from build123d import *

# Parameters (mm, degrees)
PARED_DEPTH             = 23
CONECTORES_REACH        = 154.052
CROQUIS2_W              = 16
CROQUIS2_H              = 13
CROQUIS2_W_2            = 10
CROQUIS2_H_2            = 4
BASE_START              = -1.12
BASE_FRENTE_DEPTH       = 1.12
LUCES_REACH             = 153.399
CROQUIS3_R              = 1.5
CROQUIS3_R_2            = 2.5
SALIENTE_EXTRUIR1_START = 12
CROQUIS3_3_R            = 2.3
CROQUIS3_3_R_2          = 1.5
SALIENTE_EXTRUIR1_DEPTH = 12
SALIENTE_EXTRUIR2_START = 9
CROQUIS3_4_R            = 3.3
CROQUIS3_4_R_2          = 2.5
SALIENTE_EXTRUIR2_DEPTH = 9
SALIENTE_EXTRUIR3_START = 6
CROQUIS3_5_R            = 2.3
CROQUIS3_5_R_2          = 1.5
SALIENTE_EXTRUIR3_DEPTH = 6


with BuildPart() as part:
    # Croquis1 → pared (new body)
    with BuildSketch(Plane.XY):
        with BuildLine():
            Line((3, 61.1), (132, 61.1))
            ThreePointArc((132, 61.1), (135.252691193, 59.752691193), (136.6, 56.5))
            Line((136.6, 56.5), (136.6, 3))
            ThreePointArc((136.6, 3), (135.252691193, -0.252691193), (132, -1.6))
            Line((132, -1.6), (3, -1.6))
            ThreePointArc((3, -1.6), (-0.252691193, -0.252691193), (-1.6, 3))
            Line((-1.6, 3), (-1.6, 56.5))
            ThreePointArc((-1.6, 56.5), (-0.252691193, 59.752691193), (3, 61.1))
        make_face()
        with BuildLine():
            Line((3, 0), (132, 0))
            ThreePointArc((132, 0), (134.121320344, 0.878679656), (135, 3))
            Line((135, 3), (135, 56.5))
            ThreePointArc((135, 56.5), (134.121320344, 58.621320344), (132, 59.5))
            Line((132, 59.5), (3, 59.5))
            ThreePointArc((3, 59.5), (0.878679656, 58.621320344), (0, 56.5))
            Line((0, 56.5), (0, 3))
            ThreePointArc((0, 3), (0.878679656, 0.878679656), (3, 0))
        make_face(mode=Mode.SUBTRACT)
    extrude(amount=PARED_DEPTH)

    # Croquis2 → conectores (cut, up to next)
    with BuildSketch(Plane.XZ.offset(1.6), mode=Mode.PRIVATE) as conectores_sk1:
        with Locations((110, 6.5)):
            Rectangle(CROQUIS2_W, CROQUIS2_H)
    conectores_tool1 = extrude(conectores_sk1.sketch, amount=-CONECTORES_REACH, mode=Mode.PRIVATE) & part.part
    # Croquis2 → conectores (cut, up to next)
    with BuildSketch(Plane.XZ.offset(1.6), mode=Mode.PRIVATE) as conectores_sk2:
        with Locations((95, 12)):
            Rectangle(CROQUIS2_W_2, CROQUIS2_H_2)
    conectores_tool2 = extrude(conectores_sk2.sketch, amount=-CONECTORES_REACH, mode=Mode.PRIVATE) & part.part
    add(conectores_tool1.solids().sort_by_distance((110, -1.6, 6.5))[0], mode=Mode.SUBTRACT)
    add(conectores_tool2.solids().sort_by_distance((95, -1.6, 12))[0], mode=Mode.SUBTRACT)

    # Croquis1<2> → base frente (add)
    with BuildSketch(Plane.XY.offset(BASE_START)):
        with BuildLine():
            Line((3, 61.1), (132, 61.1))
            ThreePointArc((132, 61.1), (135.252691193, 59.752691193), (136.6, 56.5))
            Line((136.6, 56.5), (136.6, 3))
            ThreePointArc((136.6, 3), (135.252691193, -0.252691193), (132, -1.6))
            Line((132, -1.6), (3, -1.6))
            ThreePointArc((3, -1.6), (-0.252691193, -0.252691193), (-1.6, 3))
            Line((-1.6, 3), (-1.6, 56.5))
            ThreePointArc((-1.6, 56.5), (-0.252691193, 59.752691193), (3, 61.1))
        make_face()
    extrude(amount=BASE_FRENTE_DEPTH)

    # Croquis3 → luces (cut, up to next)
    with BuildSketch(Plane.XY, mode=Mode.PRIVATE) as luces_sk1:
        with Locations((130.5, 48)):
            Circle(CROQUIS3_R)
    luces_tool1 = extrude(luces_sk1.sketch, amount=-LUCES_REACH, mode=Mode.PRIVATE) & part.part
    # Croquis3 → luces (cut, up to next)
    with BuildSketch(Plane.XY, mode=Mode.PRIVATE) as luces_sk2:
        with Locations((130.5, 41.5)):
            Circle(CROQUIS3_R)
    luces_tool2 = extrude(luces_sk2.sketch, amount=-LUCES_REACH, mode=Mode.PRIVATE) & part.part
    # Croquis3 → luces (cut, up to next)
    with BuildSketch(Plane.XY, mode=Mode.PRIVATE) as luces_sk3:
        with Locations((130.5, 35)):
            Circle(CROQUIS3_R)
    luces_tool3 = extrude(luces_sk3.sketch, amount=-LUCES_REACH, mode=Mode.PRIVATE) & part.part
    # Croquis3 → luces (cut, up to next)
    with BuildSketch(Plane.XY, mode=Mode.PRIVATE) as luces_sk4:
        with Locations((130.5, 28.5)):
            Circle(CROQUIS3_R)
    luces_tool4 = extrude(luces_sk4.sketch, amount=-LUCES_REACH, mode=Mode.PRIVATE) & part.part
    # Croquis3 → luces (cut, up to next)
    with BuildSketch(Plane.XY, mode=Mode.PRIVATE) as luces_sk5:
        with Locations((130.5, 17.5)):
            Circle(CROQUIS3_R)
    luces_tool5 = extrude(luces_sk5.sketch, amount=-LUCES_REACH, mode=Mode.PRIVATE) & part.part
    # Croquis3 → luces (cut, up to next)
    with BuildSketch(Plane.XY, mode=Mode.PRIVATE) as luces_sk6:
        with Locations((130.5, 11.5)):
            Circle(CROQUIS3_R_2)
    luces_tool6 = extrude(luces_sk6.sketch, amount=-LUCES_REACH, mode=Mode.PRIVATE) & part.part
    # Croquis3 → luces (cut, up to next)
    with BuildSketch(Plane.XY, mode=Mode.PRIVATE) as luces_sk7:
        with Locations((3.5, 15)):
            Circle(CROQUIS3_R)
    luces_tool7 = extrude(luces_sk7.sketch, amount=-LUCES_REACH, mode=Mode.PRIVATE) & part.part
    add(luces_tool1.solids().sort_by_distance((130.5, 48, 0))[0], mode=Mode.SUBTRACT)
    add(luces_tool2.solids().sort_by_distance((130.5, 41.5, 0))[0], mode=Mode.SUBTRACT)
    add(luces_tool3.solids().sort_by_distance((130.5, 35, 0))[0], mode=Mode.SUBTRACT)
    add(luces_tool4.solids().sort_by_distance((130.5, 28.5, 0))[0], mode=Mode.SUBTRACT)
    add(luces_tool5.solids().sort_by_distance((130.5, 17.5, 0))[0], mode=Mode.SUBTRACT)
    add(luces_tool6.solids().sort_by_distance((130.5, 11.5, 0))[0], mode=Mode.SUBTRACT)
    add(luces_tool7.solids().sort_by_distance((3.5, 15, 0))[0], mode=Mode.SUBTRACT)

    # Croquis3<3> → Saliente-Extruir1 (add)
    # profile 1 of 5: a face of its own
    with BuildSketch(Plane.XY.offset(SALIENTE_EXTRUIR1_START)):
        with Locations((130.5, 17.5)):
            Circle(CROQUIS3_3_R)
        with Locations((130.5, 17.5)):
            Circle(CROQUIS3_3_R_2, mode=Mode.SUBTRACT)
    # profile 2 of 5: a face of its own
    with BuildSketch(Plane.XY.offset(SALIENTE_EXTRUIR1_START)):
        with Locations((130.5, 28.5)):
            Circle(CROQUIS3_3_R)
        with Locations((130.5, 28.5)):
            Circle(CROQUIS3_3_R_2, mode=Mode.SUBTRACT)
    # profile 3 of 5: a face of its own
    with BuildSketch(Plane.XY.offset(SALIENTE_EXTRUIR1_START)):
        with Locations((130.5, 35)):
            Circle(CROQUIS3_3_R)
        with Locations((130.5, 35)):
            Circle(CROQUIS3_3_R_2, mode=Mode.SUBTRACT)
    # profile 4 of 5: a face of its own
    with BuildSketch(Plane.XY.offset(SALIENTE_EXTRUIR1_START)):
        with Locations((130.5, 41.5)):
            Circle(CROQUIS3_3_R)
        with Locations((130.5, 41.5)):
            Circle(CROQUIS3_3_R_2, mode=Mode.SUBTRACT)
    # profile 5 of 5: a face of its own
    with BuildSketch(Plane.XY.offset(SALIENTE_EXTRUIR1_START)):
        with Locations((130.5, 48)):
            Circle(CROQUIS3_3_R)
        with Locations((130.5, 48)):
            Circle(CROQUIS3_3_R_2, mode=Mode.SUBTRACT)
    extrude(amount=-SALIENTE_EXTRUIR1_DEPTH)

    # Croquis3<4> → Saliente-Extruir2 (add)
    with BuildSketch(Plane.XY.offset(SALIENTE_EXTRUIR2_START)):
        with Locations((130.5, 11.5)):
            Circle(CROQUIS3_4_R)
        with Locations((130.5, 11.5)):
            Circle(CROQUIS3_4_R_2, mode=Mode.SUBTRACT)
    extrude(amount=-SALIENTE_EXTRUIR2_DEPTH)

    # Croquis3<5> → Saliente-Extruir3 (add)
    with BuildSketch(Plane.XY.offset(SALIENTE_EXTRUIR3_START)):
        with Locations((3.5, 15)):
            Circle(CROQUIS3_5_R)
        with Locations((3.5, 15)):
            Circle(CROQUIS3_5_R_2, mode=Mode.SUBTRACT)
    extrude(amount=-SALIENTE_EXTRUIR3_DEPTH)


solid = part.part
Can you work these out from the model? Positions are in its coordinate system, mm. A direction names the side the tool comes from. Give positions to 0.01 mm unless a question says otherwise; leave off trailing zeros. Order: outer loops, then holes, each group sorted by start corner. A loop starts at its lowest first (then second) coordinate and runs counter-clockwise, first axis right, second up. Notation, with made-up numbers: M -0.75,-6.5 L 4.25,-6.5 A15 ccw 4.25,2.5 Z; hole C 66.25,69 d4. An arc over 180 degrees is marked long. Use a Markdown table: item, result. Add a question column.
Item 1: Suppose I cut it at B-B (x = 35). List the corners of the cut face in (y, z) for me, then the cut area to 3 significant figures.
Item 2: For faces 1 (the cylindrical face through (132.625, 16.619, 6.084)), 2 (the flat face through (67, 61.1, 11)), which set-ups out of +Z, -Z, +X, -X, +Y, -Y let a thin tool reach every point of the face, with its end or its side?
Item 3: We'd pull the mould along Y, two halves only. Please class faces 3 (the cylindrical face through (132.625, 34.119, 6.084)), 4 (the cylindrical face through (135.217, 59.788, 10.771)), 5 (the flat face through (67.8, -0.3, 23)): +Y half, -Y half, draft (parallel to the pull), parting line (faces both ways), or undercut.
Item 4: If I drill on L1, parallel to Y at x = 27, z = 10.5; L2, parallel to X at y = 43, z = 18.5; L3, parallel to X at y = 16.5, z = 10.75, over which ranges is the centre line in solid material (lowest first)? Write a range as [from, to].
Item 5: Will these pins go through, and if not, where does the flat tip stop? pin 1 (4 mm diameter, centred on x = 130.5, y = 35, fed in from +Z); pin 2 (2.5 mm diameter, centred on x = 4, y = 14.5, fed in from +Z); pin 3 (6.5 mm diameter, centred on x = 130.5, y = 11.5, fed in from +Z).
Item 6: Suppose I cut it at C-C (x = 130.5). Count the separate pieces of the cut face and the enclosed holes in it, then the cut area to 3 significant figures.
Item 7: Suppose I cut it at A-A (y = 41.5). List the corners of the cut face in (x, z) for me, then the cut area to 3 significant figures.
Answer sheet:
| question | item | result |
|---|---|---|
| 1 | outline | M -1.6,-1.12 L 61.1,-1.12 L 61.1,23 L 59.5,23 L 59.5,0 L 0,0 L 0,23 L -1.6,23 Z |
| 1 | area | 144 mm² |
| 2 | face 1 | +Z |
| 2 | face 2 | +Z, -Z, +X, -X, +Y |
| 3 | face 3 | undercut |
| 3 | face 4 | +Y half |
| 3 | face 5 | draft |
| 4 | L1 | y = [-1.6, 0], [59.5, 61.1] |
| 4 | L2 | x = [-1.6, 0], [135, 136.6] |
| 4 | L3 | x = [-1.6, 0], [128.43, 129.38], [131.62, 132.57], [135, 136.6] |
| 5 | pin 1 | stops at z = 12 |
| 5 | pin 2 | stops at z = 6 |
| 5 | pin 3 | stops at z = 9 |
| 6 | separate pieces | 7 |
| 6 | enclosed holes | 0 |
| 6 | area | 232 mm² |
| 7 | outline | M -1.6,-1.12 L 129,-1.12 L 129,12 L 128.2,12 L 128.2,0 L 0,0 L 0,23 L -1.6,23 Z; M 132,-1.12 L 136.6,-1.12 L 136.6,23 L 135,23 L 135,0 L 132.8,0 L 132.8,12 L 132,12 Z |
| 7 | area | 244 mm² |
